from build123d import *

# Parameters (mm, degrees)
SKETCH023_W     = 66
SKETCH023_H     = 61
SKETCH023_R     = 1.5
SKETCH023_R_2   = 1
SKETCH023_R_3   = 5.25
PAD016_DEPTH    = 2
SKETCH025_W     = 66
SKETCH025_H     = 61
PAD017_DEPTH    = 5
SKETCH024_R     = 5.25
SKETCH024_R_2   = 1
POCKET006_DEPTH = 3
SKETCH026_W     = 16.6
SKETCH026_H     = 24.5
POCKET007_DEPTH = 5
SKETCH029_R     = 1
POCKET009_DEPTH = 5


with BuildPart() as part:
    # Sketch023 (on DatumPlane) → Pad016 (new body)
    with BuildSketch(Plane(origin=(0, 0, -2), x_dir=(1, 0, 0), z_dir=(0, 0, -1))):
        with Locations((13, 26.5)):
            Rectangle(SKETCH023_W, SKETCH023_H)
        with Locations((-2.2, 43.75)):
            Circle(SKETCH023_R, mode=Mode.SUBTRACT)
        with Locations((2.7, 39.7)):
            Circle(SKETCH023_R_2, mode=Mode.SUBTRACT)
        with Locations((18.3, 39.7)):
            Circle(SKETCH023_R_2, mode=Mode.SUBTRACT)
        with Locations((28.2, 28.5)):
            Circle(SKETCH023_R, mode=Mode.SUBTRACT)
        with Locations((-2.2, 13.25)):
            Circle(SKETCH023_R, mode=Mode.SUBTRACT)
        with Locations((-12, 49)):
            Circle(SKETCH023_R_3, mode=Mode.SUBTRACT)
        with Locations((38, 49)):
            Circle(SKETCH023_R_3, mode=Mode.SUBTRACT)
        with Locations((-12, 4)):
            Circle(SKETCH023_R_3, mode=Mode.SUBTRACT)
        with Locations((38, 4)):
            Circle(SKETCH023_R_3, mode=Mode.SUBTRACT)
    extrude(amount=PAD016_DEPTH)

    # Sketch025 (on Face15 of Pad016) → Pad017 (join)
    with BuildSketch(Plane(origin=(0, 0, -4), x_dir=(1, 0, 0), z_dir=(0, 0, -1))):
        with Locations((13, 26.5)):
            Rectangle(SKETCH025_W, SKETCH025_H)
        Polygon((-2.838178, 47.096052), (-5.416855, 44.870347), (-4.778677, 41.524295), (-1.561822, 40.403948), (1.016855, 42.629653), (0.378677, 45.975705), align=None, mode=Mode.SUBTRACT)
        Polygon((29.500297, 25.351578), (31.576762, 28.051879), (30.276465, 31.200301), (26.899703, 31.648422), (24.823238, 28.948121), (26.123535, 25.799699), align=None, mode=Mode.SUBTRACT)
        Polygon((1.087429, 14.142269), (-1.329013, 16.543131), (-4.616442, 15.650863), (-5.487429, 12.357731), (-3.070987, 9.956869), (0.216442, 10.849137), align=None, mode=Mode.SUBTRACT)
    extrude(amount=PAD017_DEPTH)

    # Sketch024 (on Face15 of Pad016) → Pocket006 (cut)
    with BuildSketch(Plane(origin=(0, 0, -4), x_dir=(1, 0, 0), z_dir=(0, 0, -1))):
        with Locations((-12, 4)):
            Circle(SKETCH024_R)
        with Locations((-12, 49)):
            Circle(SKETCH024_R)
        with Locations((38, 49)):
            Circle(SKETCH024_R)
        with Locations((38, 4)):
            Circle(SKETCH024_R)
        with Locations((2.7, 39.7)):
            Circle(SKETCH024_R_2)
        with Locations((18.3, 39.7)):
            Circle(SKETCH024_R_2)
    extrude(amount=POCKET006_DEPTH, mode=Mode.SUBTRACT)

    # Sketch026 (on Face4 of Pocket006) → Pocket007 (cut)
    with BuildSketch(Plane.XY.offset(-2)):
        with Locations((12.5, -22.75)):
            Rectangle(SKETCH026_W, SKETCH026_H)
    extrude(amount=-POCKET007_DEPTH, mode=Mode.SUBTRACT)

    # Sketch029 (on Face4 of Pocket007) → Pocket009 (cut)
    with BuildSketch(Plane.XY.offset(-2)):
        with Locations((-2, -31.489113)):
            Circle(SKETCH029_R)
    extrude(amount=-POCKET009_DEPTH, mode=Mode.SUBTRACT)


solid = part.part
The listing builds one solid part. Answer for the finished solid, in the listing's coordinates (mm). A direction names the side the tool comes from. Give positions to 0.01 mm unless a question says otherwise; leave off trailing zeros. Write each loop counter-clockwise with the first axis right and the second up, starting at its lowest first coordinate (ties: lowest second). Pieces come first, ordered by that corner, then holes.
1) Find the intervals of material crossed by L1, parallel to X at y = -39.7, z = -4.1; L2, parallel to X at y = -49, z = -4.3; L3, parallel to Y at x = -12, z = -4.85, in increasing order.
2) Section B-B (y = -49) is taken. Write down the section's boundary in (x, z).
3) A tool of negligible diameter and unlimited length cuts with its end or side. For faces 1 (the face through (29.006, -29.765, -2.986)), 2 (the face through (30.52, -26.68, -6.46)), 3 (the face through (34.13, -52.55, -4.46)), from which of +Z, -Z, +X, -X, +Y, -Y can it reach the whole face along a straight path? Write none if from no direction.
4) For a pull along X with two mould halves and no side action, classify faces 4 (the face through (46, -26, -5)), 5 (the face through (-12, -4, -7)), 6 (the face through (13, -27, -9)) as pulls with the +X half, pulls with the -X half, needs draft (parallel to the pull), parting line crosses it, or undercut.
5) Section D-D (y = -23.5) is taken. Write down the section's boundary in (x, z), and give its area (3 significant figures).
6) Section C-C (x = -12) is taken. Write down the section's boundary in (y, z), and give its area (3 significant figures).
7) Section A-A (x = 28.2) is taken. Write down the section's boundary in (y, z).
8) Given P1, Ø1.5, axis at x = 6.5, y = -16, coming from the +Z side, flat-ended and moving along its own axis, determine where the tip first touches the part or whether it passes through.
Response:
1. L1: x = -20 to 1.7, 3.7 to 17.3, 19.3 to 46
1. L2: x = -20 to -17.25, -6.75 to 32.75, 43.25 to 46
1. L3: y = -57 to -54.25, -43.75 to -9.25, 1.25 to 4
2. outline: (-20, -9) - (46, -9) - (46, -2) - (43.25, -2) - (43.25, -7) - (32.75, -7) - (32.75, -2) - (-6.75, -2) - (-6.75, -7) - (-17.25, -7) - (-17.25, -2) - (-20, -2) - close
3. face 1: +Z, -Z
3. face 2: -Z
3. face 3: +Z
4. face 4: pulls with the +X half
4. face 5: undercut
4. face 6: needs draft
5. outline: (-20, -9) - (46, -9) - (46, -2) - (20.8, -2) - (20.8, -7) - (4.2, -7) - (4.2, -2) - (-20, -2) - close
5. area: 379 mm2
6. outline: (-57, -9) - (4, -9) - (4, -2) - (1.25, -2) - (1.25, -7) - (-9.25, -7) - (-9.25, -2) - (-43.75, -2) - (-43.75, -7) - (-54.25, -7) - (-54.25, -2) - (-57, -2) - close
6. area: 322 mm2
7. outline: (-57, -9) - (-31.48, -9) - (-31.48, -4) - (-30, -4) - (-30, -2) - (-57, -2) - close; (-27, -4) - (-25.52, -4) - (-25.52, -9) - (4, -9) - (4, -2) - (-27, -2) - close
8. P1: stops at z = -7
